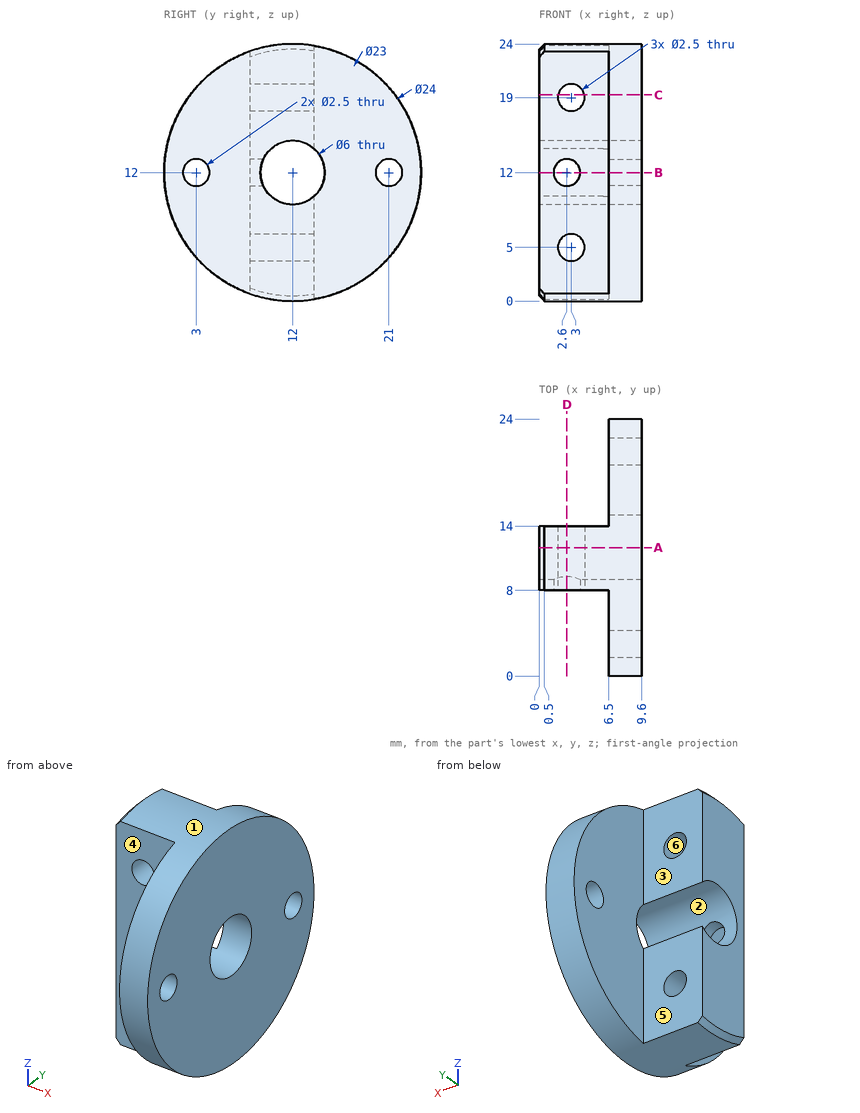
Print and shaded views of the part. All mm, measured from the part's lowest x, y and z. A direction names the side the tool comes from. Give positions to 0.01 mm unless a question says otherwise; leave off trailing zeros. Write each loop counter-clockwise with the first axis right and the second up, starting at its lowest first coordinate (ties: lowest second). Pieces come first, ordered by that corner, then holes. Notation, with made-up numbers: (47, 67.25) -> (57, 67.25) arc R19 ccw to (57, 84.25) -> close; hole circle Ø9 at (-16, 30). An arc over 180 degrees is marked (long way). Use CSV: the item, a comma, the result in double quotes. Start each with the question number.
1) Two-plate mould, pull along Z, no slides. Class the marked faces 1, 2 and 3: released by +Z, released by -Z, zero draft, split by the parting line, or undercut.
2) Pin check, flat tips, straight feed: P1, Ø4, axis at x = 3, z = 5, coming from the +Y side; P2, Ø3, axis at x = 6, z = 7, coming from the -Y side; P3, Ø1, axis at x = 8.5, y = 11, coming from the +Z side. Stop position of each tip, or through.
3) Cut at D-D on x = 2.6. List the corners of the cut face in (y, z).
4) Cut at C-C on z = 19.25. List the corners of the cut face in (x, y), plus the area to 3 significant figures.
5) Tool access for the marked faces 4, 5 and 6: list every direction of +Z, -Z, +X, -X, +Y, -Y with a clear straight run to the whole face (end or side of a thin tool).
6) Drill centre lines: L1, parallel to Y at x = 8.55, z = 12; L2, parallel to X at y = 8.7, z = 12; L3, parallel to Y at x = 8, z = 11.5. Where is each one in solid material? Low to high.
7) Cut at B-B on z = 12. List the corners of the cut face in (x, y).
8) Cut at A-A on y = 12. List the corners of the cut face in (x, z), plus the area to 3 significant figures.
Final values:
1,face 1,"split by the parting line"
1,face 2,"undercut"
1,face 3,"zero draft"
2,P1,"stops at y = 14"
2,P2,"stops at y = 0.55"
2,P3,"stops at z = 23.99"
3,outline,"(8, 0.69) arc R12 ccw to (14, 0.17) -> (14, 3.82) -> (8, 3.82) -> close; (8, 6.18) -> (14, 6.18) -> (14, 9.76) arc R3 cw to (9.27, 10.75) -> (8, 10.75) -> close; (8, 13.25) -> (9.27, 13.25) arc R3 cw to (14, 14.24) -> (14, 17.82) -> (8, 17.82) -> close; (8, 20.18) -> (14, 20.18) -> (14, 23.83) arc R12 ccw to (8, 23.31) -> close"
4,outline,"(0, 8) -> (1.78, 8) -> (1.78, 14) -> (0, 14) -> close; (4.22, 8) -> (6.5, 8) -> (6.5, 2.44) -> (9.6, 2.44) -> (9.6, 21.56) -> (6.5, 21.56) -> (6.5, 14) -> (4.22, 14) -> close"
4,area,"83.6 mm2"
5,face 4,"+Z, -Z, -X, -Y"
5,face 5,"+Z, -Z, -X, +Y"
5,face 6,"+Y, -Y"
6,L1,"y = 0 to 1.75, 4.25 to 9, 15 to 19.75, 22.25 to 24"
6,L2,"x = 0 to 1.35, 3.85 to 9.6"
6,L3,"y = 0.01 to 1.85, 4.15 to 9.04, 14.96 to 19.85, 22.15 to 23.99"
7,outline,"(0, 8) -> (1.35, 8) -> (1.35, 9) -> (0, 9) -> close; (3.85, 8) -> (6.5, 8) -> (6.5, 4.25) -> (9.6, 4.25) -> (9.6, 9) -> (3.85, 9) -> close; (6.5, 0) -> (9.6, 0) -> (9.6, 1.75) -> (6.5, 1.75) -> close; (6.5, 15) -> (9.6, 15) -> (9.6, 19.75) -> (6.5, 19.75) -> close; (6.5, 22.25) -> (9.6, 22.25) -> (9.6, 24) -> (6.5, 24) -> close"
8,outline,"(0, 0.5) -> (0.5, 0) -> (9.6, 0) -> (9.6, 9) -> (0, 9) -> close; (0, 15) -> (9.6, 15) -> (9.6, 24) -> (0.5, 24) -> (0, 23.5) -> close; hole circle Ø2.5 at (3, 5); hole circle Ø2.5 at (3, 19)"
8,area,"163 mm2"
